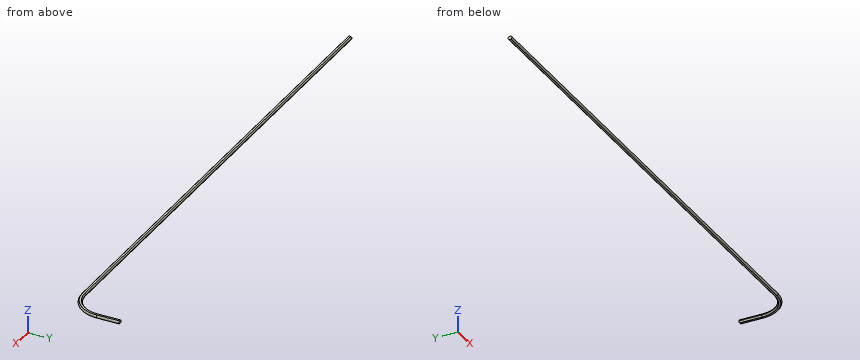
from build123d import *


with BuildPart() as f2:
    # F2: sweep along a path in F0
    with BuildLine(Plane.XY) as f2_path:
        Line((0, 0), (2720, 0))
        ThreePointArc((2720, 0), (2826.066017, 43.933983), (2870, 150))
        Line((2870, 150), (2870, 270))
    # F1 (on Right) → F2 (sweep)
    with BuildSketch(Plane.YZ):
        with BuildLine():
            ThreePointArc((5.5, -8.351647), (8.803408, -4.743416), (10, 0))
            ThreePointArc((10, 0), (8.803408, 4.743416), (5.5, 8.351647))
            Line((5.5, 8.351647), (-5.5, 8.351647))
            ThreePointArc((-5.5, 8.351647), (-10, 0), (-5.5, -8.351647))
            Line((-5.5, -8.351647), (5.5, -8.351647))
        make_face()
    sweep(path=f2_path.line)


solid = f2.part
Verification items for the finished model (mm, model axes). Give positions to 0.01 mm unless a question says otherwise; leave off trailing zeros. Write each loop counter-clockwise with the first axis right and the second up, starting at its lowest first coordinate (ties: lowest second). Pieces come first, ordered by that corner, then holes. Notation, with made-up numbers: (60, 46.25) -> (99, 46.25) arc R11 cw to (99, 52.25) -> close; hole circle Ø1 at (87, 60). An arc over 180 degrees is marked (long way). Use CSV: the item, a comma, the result in double quotes.
(1) Material ranges on L1, parallel to X at y = 126, z = -6.25; L2, parallel to Y at x = 2398, z = -4.5; L3, parallel to Y at x = 1480, z = 1.5, recorded low to high.
Derived:
L1,"x = 2860.15 to 2875.97"
L2,"y = -8.93 to 8.93"
L3,"y = -9.89 to 9.89"
(2) Sectioned sample at A-A (x = 1281). Record the cut outline in (y, z).
Derived:
outline,"(-5.5, -8.35) -> (5.5, -8.35) arc R10 ccw to (10, 0) arc R10 ccw to (5.5, 8.35) -> (-5.5, 8.35) arc R10 ccw to start"
(3) Go/stop test with flat-tipped pins: pin 1 (4 mm diameter, centred on y = 42.5, z = 1.5, fed in from -X); pin 2 (6 mm diameter, centred on y = 149.5, z = 0.5, fed in from -X); pin 3 (5 mm diameter, centred on y = 43.5, z = 6, fed in from +X). Record where each tip stops, or that it passes through.
Derived:
pin 1,"stops at x = 2807.38"
pin 2,"stops at x = 2859.96"
pin 3,"stops at x = 2839.74"
